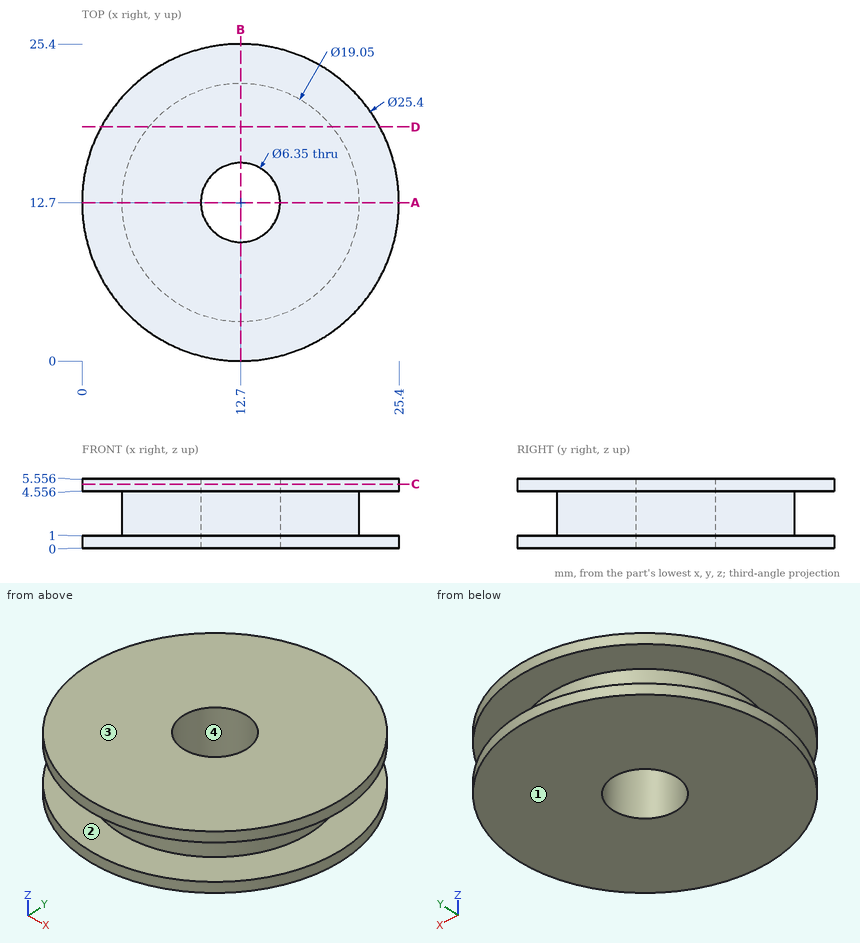
Answer from the drawing. Dimensions are ordinates in mm from the lowest x, y and z of the part. A direction names the side the tool comes from. Round coordinates to 2 decimals unless told otherwise and drop trailing zeros. Loops run counter-clockwise (first coordinate to the right, second up) from the corner with the lowest first, then second, coordinate; pieces in that order, holes last.
1) A cutting plane is placed at D-D on y = 18.75. Determine the outline of the cut face in (x, z).
Outcome:
outline: (1.53, 0) - (23.87, 0) - (23.87, 1) - (20.06, 1) - (20.06, 4.56) - (23.87, 4.56) - (23.87, 5.56) - (1.53, 5.56) - (1.53, 4.56) - (5.34, 4.56) - (5.34, 1) - (1.53, 1) - close
2) Consider line 1 (Z direction, x = 11.25, y = 22.25); line 2 (Y direction, x = 12.7, z = 2.35) (3 decimals); line 3 (X direction, y = 10.5, z = 0.9). Determine where each line is inside the solid, lowest interval first.
Outcome:
line 1: z = 0 to 1, 4.56 to 5.56
line 2: y = 3.175 to 9.525, 15.875 to 22.225
line 3: x = 0.19 to 10.41, 14.99 to 25.21
3) A cutting plane is placed at A-A on y = 12.7. Determine the outline of the cut face in (x, z) (3 decimals).
Outcome:
outline: (0, 0) - (9.525, 0) - (9.525, 5.556) - (0, 5.556) - (0, 4.556) - (3.175, 4.556) - (3.175, 1) - (0, 1) - close; (15.875, 0) - (25.4, 0) - (25.4, 1) - (22.225, 1) - (22.225, 4.556) - (25.4, 4.556) - (25.4, 5.556) - (15.875, 5.556) - close
4) For the marked faces 1 and 2, determine the directions among +Z, -Z, +X, -X, +Y, -Y from which every point of the face is accessible in a straight line to the end or side of a thin tool.
Outcome:
face 1: -Z, +X, -X, +Y, -Y
face 2: none
5) Given P1, Ø5, axis at x = 12.7, y = 12.7, coming from the -Z side; P2, Ø1, axis at x = 17.5, z = 5, coming from the +Y side; P3, Ø3, axis at y = 4, z = 3, coming from the +X side; P4, Ø2, axis at y = 8.5, z = 3, coming from the -X side, each flat-ended and moving along its own axis, determine where each tip first touches the part or whether it passes through.
Outcome:
P1: passes through
P2: stops at y = 24.65
P3: stops at x = 18.94
P4: stops at x = 3.73
6) For a pull along X with two mould halves and no side action, classify the marked faces 3 and 4 as released by +X, released by -X, zero draft, split by the parting line, or undercut.
Outcome:
face 3: zero draft
face 4: undercut
7) A cutting plane is placed at C-C on z = 5.15. Determine the outline of the cut face in (x, y) (3 decimals), plus the area to 3 significant figures.
Outcome:
outline: circle Ø25.4 at (12.7, 12.7); hole circle Ø6.35 at (12.7, 12.7)
area: 475 mm2
